For this review, take the finished solid that the model builds, in its own axes (mm). A direction names the side the tool comes from. Coordinates: 2 decimals unless noted, no trailing zeros. Order: outer loops, then holes, each group sorted by start corner. A loop starts at its lowest first (then second) coordinate and runs counter-clockwise, first axis right, second up. Notation, with made-up numbers: (-30.75, 33) - (25.25, 33) arc R26 ccw to (25.25, 53) - close; hole circle Ø10 at (57.25, -34). An arc over 180 degrees is marked (long way). One line per item, written item: value. Start each with the question number.
(1) Clearance check with flat-ended pins moving along their axes: pin 1 (12.5 mm diameter, centred on x = 10, z = 14, fed in from +Y) (3 decimals); pin 2 (1.5 mm diameter, centred on x = -0.5, y = 45.5, fed in from +Z); pin 3 (1.1 mm diameter, centred on y = 45, z = 7.5, fed in from +X). State where each tip first meets the part, or that it passes through.
(2) To check wall thickness, follow line 1 along Y through (x, z) = (-4.5, 1) (3 decimals). State the ranges of the line that lie inside material, in increasing order.
(3) Consider section B-B on z = 10.5. Write out the cut boundary in (x, y) (3 decimals).
(4) Consider section A-A on x = -4.5. Write out the cut boundary in (y, z) (3 decimals), then the cut area to 3 significant figures.
(5) For faces 1 (the flat face through (0, 46, 7)), 2 (the flat face through (0, 46, 8)), 3 (the flat face through (0, -44.095, 12)), list the 3-axis set-ups (+Z, -Z, +X, -X, +Y, -Y) from which the entire face can be reached by the end or side of a thin tool; tool diameter is ignored.
(6) Consider section C-C on x = -23.5. Write out the cut boundary in (y, z) (3 decimals).
Autodesk Inventor part; units mm, degrees
ref_plane "YZ Plane" through (0, 0, 0) normal (1, 0, 0) x (0, 1, 0)
ref_plane "XZ Plane" through (0, 0, 0) normal (0, 1, 0) x (-1, 0, 0)
ref_plane "XY Plane" through (0, 0, 0) normal (0, 0, 1) x (1, 0, 0)
sketch "Sketch2" plane through (0, 0, 0) normal (0, 0, 1) x (1, 0, 0)
  line L0 (-29.4, 44.095) -> (29.4, 44.095)
  line L1 (29.4, 44.095) -> (29.4, -44.095)
  line L2 (29.4, -44.095) -> (-29.4, -44.095)
  line L3 (-29.4, -44.095) -> (-29.4, 44.095)
  point P0 (0, 0)
  point P1 (29.4, 0)
  point P2 (0, 44.095)
  dimension "d0" = 58.8
  dimension "d1" = 88.19
extrude "Extrusion1" add sketch "Sketch2" along normal blind 25
sketch "Sketch3" plane through (-29.4, 44.095, 0) normal (0, 1, 0) x (1, 0, 0)
  line L0 (23.9, -8) -> (34.9, -8)
  line L1 (34.9, -8) -> (34.9, -7)
  line L2 (34.9, -7) -> (23.9, -7)
  line L3 (23.9, -7) -> (23.9, -8)
  line L4 (58.8, 0) -> (0, 0)
  point P0 (29.4, 0)
  point P1 (29.4, 0)
  point P2 (29.4, -7)
  dimension "d4" = 11
  dimension "d5" = 1
  dimension "d6" = 7
extrude "Extrusion2" add sketch "Sketch3" along normal blind 3
properties part number "rasberry"
Geometry check:
1. pin 1: stops at y = 44.095
1. pin 2: stops at z = 8
1. pin 3: stops at x = 5.5
2. line 1: y = -44.095 to 44.095
3. outline: (-29.4, -44.095) - (29.4, -44.095) - (29.4, 44.095) - (-29.4, 44.095) - close
4. outline: (-44.095, 0) - (44.095, 0) - (44.095, 7) - (47.095, 7) - (47.095, 8) - (44.095, 8) - (44.095, 25) - (-44.095, 25) - close
4. area: 2,210 mm^2
5. face 1: -Z, +X, -X, +Y
5. face 2: +Z, +X, -X, +Y
5. face 3: +Z, -Z, +X, -X, -Y
6. outline: (-44.095, 0) - (44.095, 0) - (44.095, 25) - (-44.095, 25) - close
